Verification items for the finished model (mm, model axes). Round coordinates to 2 decimals unless told otherwise and drop trailing zeros. Loops run counter-clockwise (first coordinate to the right, second up) from the corner with the lowest first, then second, coordinate; pieces in that order, holes last. Notation, with made-up numbers: (69.25, -35) - (93.25, -35) arc R24 ccw to (93.25, -10) - close; hole circle Ø3 at (1, 73.5). An arc over 180 degrees is marked (long way). Use CSV: the item, a comma, the result in double quotes.
```python
from build123d import *

# Parameters (mm, degrees)
BOSS_EXTRUDE1_DEPTH = 26


with BuildPart() as part:
    # Sketch1 → Boss-Extrude1 (new body)
    with BuildSketch(Plane.XY):
        with BuildLine():
            Line((0, 0), (101.5, 0))
            Line((101.5, 0), (101.5, -2))
            Line((101.5, -2), (79.678908346, -2))
            ThreePointArc((79.678908346, -2), (74, -0.5), (68.321091654, -2))
            Line((68.321091654, -2), (37.678908346, -2))
            ThreePointArc((37.678908346, -2), (32, -0.5), (26.321091654, -2))
            Line((26.321091654, -2), (0, -2))
            Line((0, -2), (0, 0))
        make_face()
    extrude(amount=BOSS_EXTRUDE1_DEPTH)


solid = part.part
```
1) Thickness scan on probe 1 along X at (y, z) = (-1.85, 16); probe 2 along X at (y, z) = (-1.7, 22); probe 3 along Y at (x, z) = (31.5, 24.5). Record the ranges inside material, lowest first. Write a range as [from, to].
Returned:
probe 1,"x = [0, 26.59], [37.41, 68.59], [79.41, 101.5]"
probe 2,"x = [0, 26.89], [37.11, 68.89], [79.11, 101.5]"
probe 3,"y = [-0.51, 0]"
2) Cross-section at A-A, the plane z = 18.25. Record the cut outline in (x, y).
Returned:
outline,"(0, -2) - (26.32, -2) arc R11.5 cw to (37.68, -2) - (68.32, -2) arc R11.5 cw to (79.68, -2) - (101.5, -2) - (101.5, 0) - (0, 0) - close"
3) Cross-section at C-C, the plane x = 78. Record the cut outline in (y, z).
Returned:
outline,"(-1.22, 0) - (0, 0) - (0, 26) - (-1.22, 26) - close"
4) Cross-section at B-B, the plane y = -1.1. Record the cut outline in (x, z), then the cut area to 3 significant figures.
Returned:
outline,"(0, 0) - (28.33, 0) - (28.33, 26) - (0, 26) - close; (35.67, 0) - (70.33, 0) - (70.33, 26) - (35.67, 26) - close; (77.67, 0) - (101.5, 0) - (101.5, 26) - (77.67, 26) - close"
area,"2,260 mm²"
5) Mould release check, pull along X, two halves, no side actions. Record for faces 1 (the face through (101.5, -1, 13)), 2 (the face through (74.1, -0.5, 12.8)), 3 (the face through (51, -1, 0)): +X half, -X half, draft (parallel to the pull), parting line (faces both ways), or undercut.
Returned:
face 1,"+X half"
face 2,"undercut"
face 3,"draft"
